Autodesk Inventor part; units mm, degrees
ref_plane "YZ Plane" through (0, 0, 0) normal (1, 0, 0) x (0, 1, 0)
ref_plane "XZ Plane" through (0, 0, 0) normal (0, 1, 0) x (-1, 0, 0)
ref_plane "XY Plane" through (0, 0, 0) normal (0, 0, 1) x (1, 0, 0)
sketch "Sketch1" plane through (0, 0, 0) normal (0, 1, 0) x (-1, 0, 0)
  line L0 (-17.05, 12.2) -> (17.05, 12.2)
  line L1 (17.05, 12.2) -> (17.05, -12.2)
  line L2 (17.05, -12.2) -> (-17.05, -12.2)
  line L3 (-17.05, -12.2) -> (-17.05, 12.2)
  line L4 (-17.05, 12.2) -> (17.05, -12.2) construction
  line L5 (17.05, 12.2) -> (-17.05, -12.2) construction
  point P0 (0, 0)
  dimension "d0" = 34.1
  dimension "d1" = 24.4
extrude "Extrusion1" add sketch "Sketch1" along normal blind 1.6
sketch "Sketch2" plane through (0, 1.6, 0) normal (0, 1, 0) x (1, 0, 0)
  circle A0 centre (-14.92, -10) radius 1.5
  circle A1 centre (-14.92, 10) radius 1.5
  line L0 (-17.05, 12.2) -> (-17.05, -12.2)
  line L1 (-17.05, -12.2) -> (17.05, -12.2)
  line L2 (17.05, 12.2) -> (-17.05, 12.2)
  circle A2 centre (14.26, -6.35) radius 0.4
  circle A3 centre (14.26, -3.81) radius 0.4
  circle A4 centre (14.26, -1.27) radius 0.4
  circle A5 centre (14.26, -8.89) radius 0.4
  circle A6 centre (14.26, 1.27) radius 0.4
  line L3 (17.05, -12.2) -> (17.05, 12.2)
  circle A7 centre (14.26, 3.81) radius 0.4
  circle A8 centre (14.26, 6.35) radius 0.4
  circle A9 centre (14.26, 8.89) radius 0.4
  point P0 (0, 0)
  dimension "d4" = 3
  dimension "d5" = 3
  dimension "d6" = 2.13
  dimension "d7" = 2.2
  dimension "d8" = 2.13
  dimension "d9" = 2.2
  dimension "d10" = 0.8
  dimension "d11" = 0.8
  dimension "d12" = 2.54
  dimension "d13" = 0.8
  dimension "d14" = 0.8
  dimension "d15" = 0.8
  dimension "d16" = 2.79
  dimension "d17" = 2.54
  dimension "d18" = 2.79
  dimension "d19" = 2.79
  dimension "d20" = 2.79
  dimension "d21" = 2.54
  dimension "d22" = 2.79
  dimension "d23" = 2.54
  dimension "d24" = 0.8
  dimension "d25" = 0.8
  dimension "d26" = 0.8
  dimension "d27" = 2.79
  dimension "d28" = 2.79
  dimension "d29" = 2.79
  dimension "d30" = 2.54
  dimension "d31" = 2.54
  dimension "d32" = 2.54
  dimension "d33" = 3.31
extrude "Extrusion2" cut sketch "Sketch2" against normal blind 3.31 contours A0 | A1 | A2 | A3 | A4 | A5 | A6 | A7 | A8 | A9
sketch "Sketch3" plane through (0, 1.6, 0) normal (0, 1, 0) x (1, 0, 0)
  line L0 (-16.05, -7.5) -> (-1.05, -7.5)
  line L1 (-1.05, -7.5) -> (-1.05, 7.5)
  line L2 (-1.05, 7.5) -> (-16.05, 7.5)
  line L3 (-16.05, 7.5) -> (-16.05, -7.5)
  line L4 (-16.05, -7.5) -> (-1.05, 7.5) construction
  line L5 (-1.05, -7.5) -> (-16.05, 7.5) construction
  line L6 (-17.05, 12.2) -> (-17.05, -12.2)
  point P0 (0, 0)
  point P1 (-8.55, 0)
  dimension "d36" = 15
  dimension "d37" = 15
  dimension "d38" = 1
extrude "Extrusion3" add sketch "Sketch3" along normal blind 3.3
equation "\"d34\" = d33"
properties part number "arducam'"
For this review, take the finished solid that the model builds, in its own axes (mm). A direction names the side the tool comes from. Round coordinates to 2 decimals unless told otherwise and drop trailing zeros. Write each loop counter-clockwise with the first axis right and the second up, starting at its lowest first coordinate (ties: lowest second). Pieces come first, ordered by that corner, then holes. Notation, with made-up numbers: (55.25, -2) - (81.25, -2) arc R16 cw to (81.25, 7) - close; hole circle Ø5 at (8, 74). An arc over 180 degrees is marked (long way). Use CSV: the item, a comma, the result in double quotes.
1) The part is to be moulded in two halves that separate along X. For faces 1 (the cylindrical face through (14.445, 0.811, 9.245)), 2 (the flat face through (-8, 3, -7.5)), 3 (the flat face through (-17.05, 1, 0)), say which applies: pulls with the +X half, pulls with the -X half, needs draft (parallel to the pull), parting line crosses it, or undercut.
Conclusion:
face 1,"undercut"
face 2,"needs draft"
face 3,"pulls with the -X half"
2) Add section C-C on x = -6. Write out the cut boundary in (y, z), and give its area (3 significant figures).
Conclusion:
outline,"(0, -12.2) - (1.6, -12.2) - (1.6, -7.5) - (4.9, -7.5) - (4.9, 7.5) - (1.6, 7.5) - (1.6, 12.2) - (0, 12.2) - close"
area,"88.5 mm^2"
3) Wall thickness on line 1 along X through (y, z) = (1.3, -1.27); line 2 along Y through (x, z) = (8, 2.5); line 3 along X through (y, z) = (3.5, -3): over which ranges is each line inside the solid? List them lowest first. Write a range as from..to.
Conclusion:
line 1,"x = -17.05..13.86, 14.66..17.05"
line 2,"y = 0..1.6"
line 3,"x = -16.05..-1.05"
4) Add section B-B on y = 1.15. Count the separate pieces of the cut face and the enclosed holes in it, and give its area (3 significant figures).
Conclusion:
separate pieces,"1"
enclosed holes,"10"
area,"814 mm^2"
5) Add section D-D on z = -8.89. Write out the cut boundary in (x, y), and give its area (3 significant figures).
Conclusion:
outline,"(-17.05, 0) - (-15.93, 0) - (-15.93, 1.6) - (-17.05, 1.6) - close; (-13.91, 0) - (13.86, 0) - (13.86, 1.6) - (-13.91, 1.6) - close; (14.66, 0) - (17.05, 0) - (17.05, 1.6) - (14.66, 1.6) - close"
area,"50.1 mm^2"
6) For faces 4 (the flat face through (-9, 3, 7.5)), 5 (the flat face through (-1.05, 3, 0)), 6 (the flat face through (-16.05, 3, 0)), list the 3-axis set-ups (+Z, -Z, +X, -X, +Y, -Y) from which the entire face can be reached by the end or side of a thin tool; tool diameter is ignored.
Conclusion:
face 4,"+Z, +X, -X, +Y"
face 5,"+Z, -Z, +X, +Y"
face 6,"+Z, -Z, -X, +Y"
7) Clearance check with flat-ended pins moving along their axes: pin 1 Ø6 at (x, z) = (-6, 9) entering from -Y; pin 2 Ø1.6 at (y, z) = (3.5, 1.5) entering from -X; pin 3 Ø4 at (x, z) = (-14.92, -10) entering from +Y; pin 4 Ø1 at (x, y) = (-10.5, 3) entering from -Z. State where each tip first meets the part, or that it passes through.
Conclusion:
pin 1,"stops at y = 0"
pin 2,"stops at x = -16.05"
pin 3,"stops at y = 1.6"
pin 4,"stops at z = -7.5"
8) Add section A-A on z = -6.35. Write out the cut boundary in (x, y).
Conclusion:
outline,"(-17.05, 0) - (13.86, 0) - (13.86, 1.6) - (-1.05, 1.6) - (-1.05, 4.9) - (-16.05, 4.9) - (-16.05, 1.6) - (-17.05, 1.6) - close; (14.66, 0) - (17.05, 0) - (17.05, 1.6) - (14.66, 1.6) - close"
